Build history of the part. All positions in model axes, mm. Face numbers are marked on the shaded views. A direction names the side the tool comes from. Round coordinates to 2 decimals unless told otherwise and drop trailing zeros. Write each loop counter-clockwise with the first axis right and the second up, starting at its lowest first coordinate (ties: lowest second). Pieces come first, ordered by that corner, then holes.
1) Flat gauge pins, fed straight in: pin 1 (10 mm diameter, centred on x = -11, z = -14, fed in from -Y); pin 2 (6.5 mm diameter, centred on x = -63, z = 23, fed in from +Y); pin 3 (10 mm diameter, centred on y = 40, z = -4, fed in from -X). Where does each tip first touch, or does it go through?
2) Saw through at A-A (y = 78.5). Write the cut outline in (x, z).
3) Pull direction Y, two halves, no side cores. Call the marked faces 1, 2 and 3: +Y half, -Y half, draft (parallel to the pull), parting line (faces both ways), or undercut.
4) Which spindle directions (+Z, -Z, +X, -X, +Y, -Y) get a long thin tool onto all of the face, cutting with end or side? Do the marked faces 4, 5 and 6. Say none if no direction does.
5) Saw through at D-D (x = 11). Write the cut outline in (y, z), plus the area to 3 significant figures.
6) Saw through at B-B (x = -63). Write the cut outline in (y, z).
7) Wall check: probe 1 along X at (y, z) = (4, -23); probe 2 along Z at (x, y) = (-63, 3.55); probe 3 along Y at (x, z) = (24.5, 25). Give the ranges that are in metal, low to high.
8) Saw through at C-C (z = -16.5). Write the cut outline in (x, y).
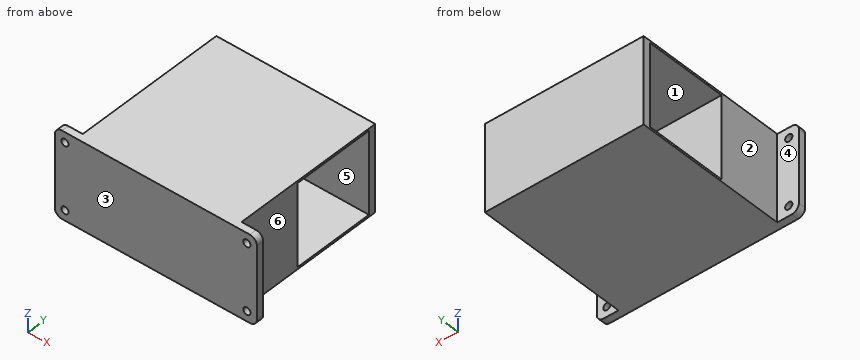
from build123d import *

# Parameters (mm, degrees)
SKETCH_1_W          = 140
SKETCH_1_H          = 60
EXTRUDE_3_DEPTH     = 5
SKETCH_3_W          = 110
SKETCH_3_H          = 60
EXTRUDE_4_DEPTH     = 106.5
FILLET_1_R          = 5
SKETCH_19_W         = 57
SKETCH_19_H         = 57
CUT_EXTRUDE_1_DEPTH = 160
HOLE_WIZARD_M6_2_D  = 5


with BuildPart() as part:
    # 草图1 → 凸台-拉伸3 (new body)
    with BuildSketch(Plane(origin=(0, 0, 0), x_dir=(1, 0, 0), z_dir=(0, 1, 0))):
        Rectangle(SKETCH_1_W, SKETCH_1_H)
    extrude(amount=EXTRUDE_3_DEPTH)

    # 草图3 → 凸台-拉伸4 (add)
    with BuildSketch(Plane(origin=(0, 5, 0), x_dir=(1, 0, 0), z_dir=(0, 1, 0))):
        Rectangle(SKETCH_3_W, SKETCH_3_H)
    extrude(amount=EXTRUDE_4_DEPTH)

    # 圆角1
    fillet_1_edges = [part.edges().sort_by_distance(p)[0] for p in [
        (70, 2.5, 30),
        (-70, 2.5, 30),
        (-70, 2.5, -30),
        (70, 2.5, -30),
    ]]
    fillet(fillet_1_edges, radius=FILLET_1_R)

    # 草图19 → 切除-拉伸1 (cut)
    with BuildSketch(Plane.ZY.offset(55)):
        with Locations((0, 78)):
            Rectangle(SKETCH_19_W, SKETCH_19_H)
    extrude(amount=-CUT_EXTRUDE_1_DEPTH, mode=Mode.SUBTRACT)

    # M6 螺纹孔2 (through all)
    with Locations(Plane(origin=(0, 5, 0), x_dir=(1, 0, 0), z_dir=(0, 1, 0))):
        with Locations((-63, 23), (63, 23), (63, -23), (-63, -23)):
            Hole(HOLE_WIZARD_M6_2_D / 2)


solid = part.part
Evaluation:
1. pin 1: stops at y = 0
1. pin 2: stops at y = 5
1. pin 3: stops at x = -55
2. outline: (-55, -30) - (55, -30) - (55, -28.5) - (-55, -28.5) - close; (-55, 28.5) - (55, 28.5) - (55, 30) - (-55, 30) - close
3. face 1: undercut
3. face 2: draft
3. face 3: -Y half
4. face 4: +Z, -Z, -X, +Y
4. face 5: +X, -X
4. face 6: +Z, -Z, +X, +Y
5. outline: (0, -30) - (111.5, -30) - (111.5, 30) - (0, 30) - close; hole (49.5, -28.5) - (106.5, -28.5) - (106.5, 28.5) - (49.5, 28.5) - close
5. area: 3,440 mm2
6. outline: (0, -30) - (5, -30) - (5, -25.5) - (0, -25.5) - close; (0, -20.5) - (5, -20.5) - (5, 20.5) - (0, 20.5) - close; (0, 25.5) - (5, 25.5) - (5, 30) - (0, 30) - close
7. probe 1: x = -70 to -65.5, -60.5 to 60.5, 65.5 to 70
7. probe 2: z = -30 to -25.5, -20.5 to 20.5, 25.5 to 30
7. probe 3: y = 0 to 49.5, 106.5 to 111.5
8. outline: (-70, 0) - (70, 0) - (70, 5) - (55, 5) - (55, 49.5) - (-55, 49.5) - (-55, 5) - (-70, 5) - close; (-55, 106.5) - (55, 106.5) - (55, 111.5) - (-55, 111.5) - close
